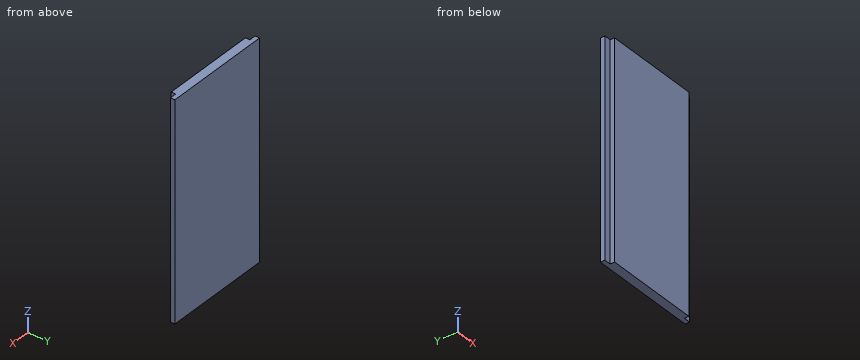
Autodesk Inventor part; units mm, degrees
ref_plane "YZ Plane" through (0, 0, 0) normal (1, 0, 0) x (0, 1, 0)
ref_plane "XZ Plane" through (0, 0, 0) normal (0, 1, 0) x (-1, 0, 0)
ref_plane "XY Plane" through (0, 0, 0) normal (0, 0, 1) x (1, 0, 0)
sketch "Skizze1" plane through (0, 0, 0) normal (0, 0, 1) x (1, 0, 0)
  line L0 (73, -6) -> (-73, -6)
  line L1 (-73, -6) -> (-73, 6)
  line L2 (-73, 6) -> (73, 6)
  line L3 (73, 6) -> (73, -6)
  line L4 (73, -6) -> (-73, 6) construction
  line L5 (-73, -6) -> (73, 6) construction
  point P0 (0, 0)
  dimension "d0" = 146
  dimension "d1" = 12
extrude "Extrusion1" add sketch "Skizze1" along normal blind 289
sketch "Skizze2" plane through (0, 0, 0) normal (0, 0, -1) x (-1, 0, 0)
  line L0 (-73, -6) -> (-64, -6)
  line L1 (-64, -6) -> (-64, 0)
  line L2 (-64, 0) -> (-73, 0)
  line L3 (-73, 0) -> (-73, -6)
  line L4 (73, -6) -> (64, -6)
  line L5 (64, -6) -> (64, 0)
  line L6 (64, 0) -> (73, 0)
  line L7 (73, 0) -> (73, -6)
  point P0 (0, 0)
  dimension "d4" = 6
  dimension "d5" = 128
  dimension "d6" = 64
extrude "Extrusion2" cut sketch "Skizze2" against normal through all
properties part number "Lid_MaintenanceCover" material "Polycarbonat, klar"
Can you work these out from the model? Positions are in its coordinate system, mm. Coordinates: 2 decimals unless noted, no trailing zeros. Order: outer loops, then holes, each group sorted by start corner. A loop starts at its lowest first (then second) coordinate and runs counter-clockwise, first axis right, second up. Notation, with made-up numbers: (-1.5, 30) - (11.5, 30) arc R26 cw to (11.5, 52) - close; hole circle Ø8 at (55, 11.25). An arc over 180 degrees is marked (long way). Answer as a JSON object with one key per item and string values. Group by question number.
Q1. Will these pins go through, and if not, where does the flat tip stop? P1, Ø1.8, axis at y = -3, z = 161, coming from the +X side; P2, Ø4.5, axis at x = 68.5, z = 208.5, coming from the -Y side; P3, Ø3, axis at y = -2, z = 184.5, coming from the -X side.
Q2. I need wall thicknesses on line 1 (X direction, y = -0.25, z = 76). Which ranges of the line are inside material? Lowest first, please. Write a range as from..to.
Q3. Imagine slicing it at A-A (z = 43.5). Please give me the cut outline in (x, y).
Q4. Imagine slicing it at B-B (y = -2). Please give me the cut outline in (x, z), and give its area (3 significant figures).
Determined:
{
 "1": {"P1": "stops at x = 64", "P2": "stops at y = 0", "P3": "stops at x = -64"},
 "2": {"line 1": "x = -64..64"},
 "3": {"outline": "(-73, 0) - (-64, 0) - (-64, -6) - (64, -6) - (64, 0) - (73, 0) - (73, 6) - (-73, 6) - close"},
 "4": {"outline": "(-64, 0) - (64, 0) - (64, 289) - (-64, 289) - close", "area": "37,000 mm2"}
}
